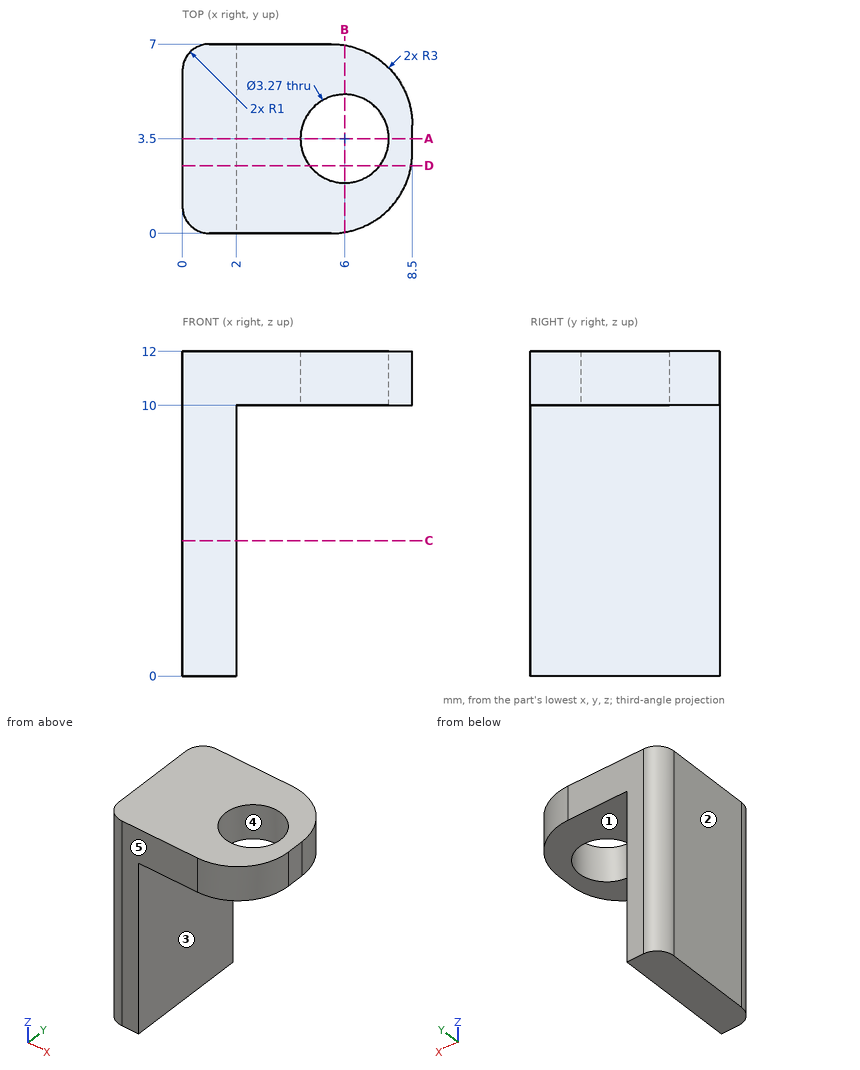
Verification items for this drawing (mm, ordinates from the low corner). A direction names the side the tool comes from. Round coordinates to 2 decimals unless told otherwise and drop trailing zeros. Write each loop counter-clockwise with the first axis right and the second up, starting at its lowest first coordinate (ties: lowest second). Pieces come first, ordered by that corner, then holes. Notation, with made-up numbers: (4, -19.75) - (53, -19.75) arc R16 ccw to (53, 4.25) - close; hole circle Ø11 at (65, 83.5). An arc over 180 degrees is marked (long way). Answer as a JSON object with one key per item and string values. Group by question number.
Q1. Section check B-B, the plane x = 6. Enter the section's corners in (y, z) (3 decimals).
Q2. Thickness scan on line 1 (X direction, y = 2.25, z = 6.75); line 2 (X direction, y = 3.75, z = 10.75); line 3 (Y direction, x = 6, z = 10.85) (3 decimals). Record the ranges inside material, lowest first.
Q3. Tool access check on the marked faces 1 and 2. Record the directions out of +Z, -Z, +X, -X, +Y, -Y that give a thin tool (end or side, any length) a straight path to the whole face; none if there is none.
Q4. Section check D-D, the plane y = 2.5. Enter the section's corners in (x, z).
Q5. Go/stop test with a flat-tipped pin: pin 1 Ø1 at (y, z) = (4.5, 4) entering from +X. Record where the tip stops, or that it passes through.
Q6. Section check C-C, the plane z = 5. Enter the section's corners in (x, y).
Q7. Mould release check, pull along Y, two halves, no side actions. Record for the marked faces 3, 4 and 5: released by +Y, released by -Y, zero draft, split by the parting line, or undercut.
Q8. Section check A-A, the plane y = 3.5. Enter the section's corners in (x, z) (3 decimals).
Found:
{
 "1": {"outline": "(0.042, 10) - (1.865, 10) - (1.865, 12) - (0.042, 12) - close; (5.135, 10) - (6.958, 10) - (6.958, 12) - (5.135, 12) - close"},
 "2": {"line 1": "x = 0 to 2", "line 2": "x = 0 to 4.38, 7.62 to 8.5", "line 3": "y = 0.042 to 1.865, 5.135 to 6.958"},
 "3": {"face 1": "-Z, +X, +Y, -Y", "face 2": "+Z, -Z, -X, +Y, -Y"},
 "4": {"outline": "(0, 0) - (2, 0) - (2, 10) - (4.71, 10) - (4.71, 12) - (0, 12) - close; (7.29, 10) - (8.46, 10) - (8.46, 12) - (7.29, 12) - close"},
 "5": {"pin 1": "stops at x = 2"},
 "6": {"outline": "(0, 1) arc R1 ccw to (1, 0) - (2, 0) - (2, 7) - (1, 7) arc R1 ccw to (0, 6) - close"},
 "7": {"face 3": "zero draft", "face 4": "undercut", "face 5": "released by -Y"},
 "8": {"outline": "(0, 0) - (2, 0) - (2, 10) - (4.365, 10) - (4.365, 12) - (0, 12) - close; (7.635, 10) - (8.5, 10) - (8.5, 12) - (7.635, 12) - close"}
}
